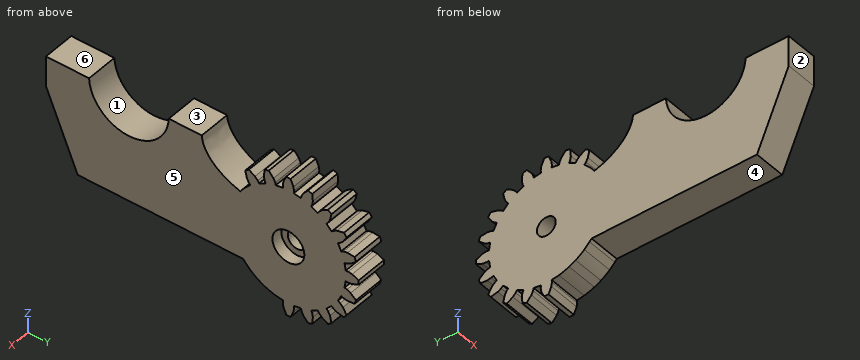
```python
from build123d import *

# Parameters (mm, degrees)
BOSS_EXTRUDE1_DEPTH = 10
SKETCH3_R           = 2.95
CUT_EXTRUDE1_DEPTH  = 10
CUT_EXTRUDE4_DEPTH  = 10
BOSS_EXTRUDE2_DEPTH = 10
SKETCH9_R           = 5
CUT_EXTRUDE5_DEPTH  = 3.5


with BuildPart() as part:
    # Sketch1 → Boss-Extrude1 (new body)
    with BuildSketch(Plane.YZ):
        Polygon((122.8604, 156.33104), (123.6529, 156.40531), (124.8827, 156.22038), (126.9389, 155.34362), (126.9389, 153.95038), (124.8827, 153.07362), (123.6529, 152.88869), (122.8604, 152.96296), (122.5013, 150.69576), (123.278, 150.5215), (124.3904, 149.9656), (126.075, 148.49636), (125.6445, 147.1713), (123.418, 146.97285), (122.1913, 147.17699), (121.4605, 147.49252), (120.4184, 145.44725), (121.1032, 145.04152), (121.9894, 144.1691), (123.1376, 142.2512), (122.3186, 141.124), (120.1398, 141.6233), (119.0362, 142.1965), (118.4387, 142.7224), (116.8156, 141.0993), (117.3415, 140.5018), (117.9147, 139.3982), (118.414, 137.2194), (117.2868, 136.4004), (115.3689, 137.5486), (114.49648, 138.4348), (114.09075, 139.1196), (112.04548, 138.0775), (112.36101, 137.3467), (112.56515, 136.12), (112.3667, 133.8935), (111.04164, 133.463), (109.5724, 135.1476), (109.0165, 136.26), (108.84224, 137.0367), (106.57504, 136.6776), (106.64931, 135.8851), (106.46438, 134.6553), (105.58762, 132.5991), (104.19438, 132.5991), (103.31762, 134.6553), (103.13269, 135.8851), (103.20696, 136.6776), (100.93976, 137.0367), (100.7655, 136.26), (100.2096, 135.1476), (98.74036, 133.463), (97.4153, 133.8935), (97.21685, 136.12), (97.42099, 137.3467), (97.73652, 138.0775), (95.69125, 139.1196), (95.28552, 138.4348), (94.4131, 137.5486), (92.4952, 136.4004), (91.368, 137.2194), (91.8673, 139.3982), (92.4405, 140.5018), (92.9664, 141.0993), (91.3433, 142.7224), (90.7458, 142.1965), (89.6422, 141.6233), (87.4634, 141.124), (86.6444, 142.2512), (87.7926, 144.1691), (88.6788, 145.04152), (89.3636, 145.44725), (88.3215, 147.49252), (87.5907, 147.17699), (86.364, 146.97285), (84.1375, 147.1713), (83.707, 148.49636), (85.3916, 149.9656), (86.504, 150.5215), (87.2807, 150.69576), (86.9216, 152.96296), (86.1291, 152.88869), (84.8993, 153.07362), (82.8431, 153.95038), (82.8431, 155.34362), (84.8993, 156.22038), (86.1291, 156.40531), (86.9216, 156.33104), (87.2807, 158.59824), (86.504, 158.7725), (85.3916, 159.3284), (83.707, 160.79764), (84.1375, 162.1227), (86.364, 162.32115), (87.5907, 162.11701), (88.3215, 161.80148), (89.3636, 163.84675), (88.6788, 164.25248), (87.7926, 165.1249), (86.6444, 167.0428), (87.4634, 168.17), (89.6422, 167.6707), (90.7458, 167.0975), (91.3433, 166.5716), (92.9664, 168.1947), (92.4405, 168.7922), (91.8673, 169.8958), (91.368, 172.0746), (92.4952, 172.8936), (94.4131, 171.7454), (95.28552, 170.8592), (95.69125, 170.1744), (97.73652, 171.2165), (97.42099, 171.9473), (97.21685, 173.174), (97.4153, 175.4005), (98.74036, 175.831), (100.2096, 174.1464), (100.7655, 173.034), (100.93976, 172.2573), (103.20696, 172.6164), (103.13269, 173.4089), (103.31762, 174.6387), (104.19438, 176.6949), (105.58762, 176.6949), (106.46438, 174.6387), (106.64931, 173.4089), (106.57504, 172.6164), (108.84224, 172.2573), (109.0165, 173.034), (109.5724, 174.1464), (111.04164, 175.831), (112.3667, 175.4005), (112.56515, 173.174), (112.36101, 171.9473), (112.04548, 171.2165), (114.09075, 170.1744), (114.49648, 170.8592), (115.3689, 171.7454), (117.2868, 172.8936), (118.414, 172.0746), (117.9147, 169.8958), (117.3415, 168.7922), (116.8156, 168.1947), (118.4387, 166.5716), (119.0362, 167.0975), (120.1398, 167.6707), (122.3186, 168.17), (123.1376, 167.0428), (121.9894, 165.1249), (121.1032, 164.25248), (120.4184, 163.84675), (121.4605, 161.80148), (122.1913, 162.11701), (123.418, 162.32115), (125.6445, 162.1227), (126.075, 160.79764), (124.3904, 159.3284), (123.278, 158.7725), (122.5013, 158.59824), align=None)
    extrude(amount=BOSS_EXTRUDE1_DEPTH)

    # Sketch3 → Cut-Extrude1 (cut)
    with BuildSketch(Plane.YZ.offset(10)):
        with Locations(Location((104.891, 154.647, 0), (0, 0, 270))):
            Circle(SKETCH3_R)
    extrude(amount=-CUT_EXTRUDE1_DEPTH, mode=Mode.SUBTRACT)

    # Sketch5 → Cut-Extrude4 (cut)
    with BuildSketch(Plane.YZ.offset(10)):
        with BuildLine():
            Line((100.93976, 137.0367), (100.054261516, 133.090117674))
            ThreePointArc((100.054261516, 133.090117674), (83.487848916, 149.169926106), (90.294048938, 171.230794333))
            Line((90.294048938, 171.230794333), (92.9664, 168.1947))
            ThreePointArc((92.9664, 168.1947), (87.406270735, 150.172651628), (100.93976, 137.0367))
        make_face()
    extrude(amount=-CUT_EXTRUDE4_DEPTH, mode=Mode.SUBTRACT)


with BuildPart() as cut_extrude4_kept_piece:
    # of the separate pieces the step leaves, the one the design keeps (cut_extrude4_pieces_kept)
    add(part.part.solids().sort_by_distance((0, 122.8604, 156.33104))[0])

    # Sketch8 → Boss-Extrude2 (add)
    with BuildSketch(Plane(origin=(0, 0, 0), x_dir=(0, -1, 0), z_dir=(-1, 0, 0))):
        with BuildLine():
            Line((-98.898724503, 146.469883253), (-98.898724503, 143.469883253))
            Line((-98.898724503, 143.469883253), (-38.832437603, 143.469883253))
            Line((-38.832437603, 143.469883253), (-28.891, 166.6949))
            Line((-28.891, 166.6949), (-28.891, 176.1949))
            Line((-28.891, 176.1949), (-42.401004003, 176.1949))
            ThreePointArc((-42.401004003, 176.1949), (-54.891, 164.1949), (-67.380995997, 176.1949))
            Line((-67.380995997, 176.1949), (-77.731516388, 176.1949))
            add(Edge.make_bspline(
                [(-98.898724503, 163.298263053), (-78.493111017, 163.298263053), (-77.731516388, 176.1949)],
                knots=[1.570796327, 1.570796327, 1.570796327, 3.104261183, 3.104261183, 3.104261183], degree=2, weights=[1, 0.720181505, 1]))
            Line((-98.898724503, 163.298263053), (-98.898724503, 146.469883253))
        make_face()
    extrude(amount=-BOSS_EXTRUDE2_DEPTH)

    # Sketch9 → Cut-Extrude5 (cut)
    with BuildSketch(Plane.YZ.offset(10)):
        with Locations(Location((104.891, 154.647, 0), (0, 0, 270))):
            Circle(SKETCH9_R)
    extrude(amount=-CUT_EXTRUDE5_DEPTH, mode=Mode.SUBTRACT)


solid = cut_extrude4_kept_piece.part
```
Check sheet for the modelled part. Datum: model origin and axes. Units: mm. Face numbers are marked on the shaded views. A direction names the side the tool comes from. Coordinates: 2 decimals unless noted, no trailing zeros. Write each loop counter-clockwise with the first axis right and the second up, starting at its lowest first coordinate (ties: lowest second). Pieces come first, ordered by that corner, then holes. Notation, with made-up numbers: M -21.5,78 L 16.5,78 A4 ccw 16.5,83 Z; hole C -22,37.5 d5. An arc over 180 degrees is marked long. Use one line per item in the form item = value.
Item 1: Set-up check for the marked faces 4, 5 and 6: record each of +Z, -Z, +X, -X, +Y, -Y from which the full face is reachable in a straight line by a thin tool's end or side.
Answer below:
face_4 = -Z, +X, -X, -Y
face_5 = +Z, -Z, +X, +Y, -Y
face_6 = +Z, +X, -X, -Y
Item 2: Gauge pin test, flat ends, axial feed: pin 1 Ø3 at (x, y) = (6.5, 52) entering from -Z; pin 2 Ø5.5 at (y, z) = (104.891, 154.647) entering from -X; pin 3 Ø6 at (x, z) = (1, 148) entering from -Y; pin 4 Ø5 at (x, y) = (4, 72.5) entering from +Z. Record the tip position at first contact, or that the pin passes through.
Answer below:
pin_1 = 143.47
pin_2 = through
pin_3 = 35.61
pin_4 = 176.19
Item 3: Material ranges on L1, parallel to Y at x = 3, z = 166.5; L2, parallel to Y at x = 9, z = 173; L3, parallel to Y at x = 6.5, z = 167, recorded low to high. Write a range as from..to.
Answer below:
L1 = 28.97..47.66, 62.12..85.16, 91.28..122.81
L2 = 28.89..42.95, 66.83..78.54, 97.25..100.77, 103.17..106.61, 109.01..112.54
L3 = 28.89..47, 62.78..84.28, 91.77..118.01, 118.93..123.11
Item 4: Release check for a two-part mould opening along Y. For the marked faces 1, 2 and 3 record: pulls with the +Y half, pulls with the -Y half, needs draft (parallel to the pull), parting line crosses it, or undercut.
Answer below:
face_1 = undercut
face_2 = pulls with the -Y half
face_3 = needs draft
Item 5: Sectioned sample at A-A, the plane y = 76.5. Record the cut outline in (x, z), and give its area (3 significant figures).
Answer below:
outline = M 0,143.47 L 10,143.47 L 10,176.19 L 0,176.19 Z
area = 327 mm^2
Item 6: Sectioned sample at B-B, the plane y = 49.5. Record the cut outline in (x, z).
Answer below:
outline = M 0,143.47 L 10,143.47 L 10,165.42 L 0,165.42 Z
